The model under review builds one solid part; all positions refer to its coordinate system, in mm. Round coordinates to 2 decimals unless told otherwise and drop trailing zeros. Write each loop counter-clockwise with the first axis right and the second up, starting at its lowest first coordinate (ties: lowest second). Pieces come first, ordered by that corner, then holes. Notation, with made-up numbers: (-15, 3.25) -> (20, 3.25) arc R18 ccw to (20, 29.25) -> close; hole circle Ø1 at (-21, 54.25). An arc over 180 degrees is marked (long way). Return JSON: item names as keys, results as strings. Group by question number.
1. Clearance check with flat-ended pins moving along their axes: P1, Ø1.5, axis at x = -53, z = 4.5, coming from the +Y side; P2, Ø3, axis at x = 20.5, z = 9, coming from the +Y side; P3, Ø3, axis at y = -53, z = 6.5, coming from the +X side. State where each tip first meets the part, or that it passes through.
2. Take a section at B-B, the plane y = 5. Write out the cut boundary in (x, z).
3. Take a section at D-D, the plane x = 5. Write out the cut boundary in (y, z), then the cut area to 3 significant figures.
4. Take a section at A-A, the plane x = -52.5. Write out the cut boundary in (y, z), then the cut area to 3 significant figures.
5. Take a section at C-C, the plane y = -51. Write out the cut boundary in (x, z).
6. For line 1 along X through (y, z) = (42.5, 5); line 2 along X through (y, z) = (0.5, 4.75); line 3 along Z through (x, y) = (52.5, -45.25), list the stretches that pass through material, from the lowest coordinate up. Write a range as from..to.
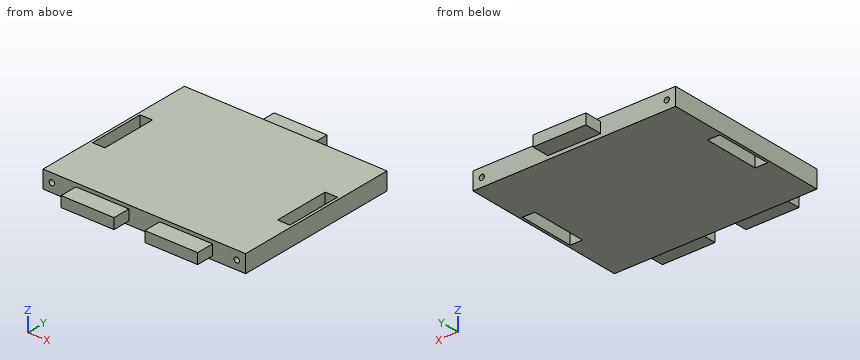
from build123d import *

# Parameters (mm, degrees)
ESBO_O1_W                = 115
ESBO_O1_H                = 95
RESSALTO_EXTRUS_O1_DEPTH = 10
ESBO_O2_W                = 30
ESBO_O2_H                = 6
RESSALTO_EXTRUS_O2_DEPTH = 10
ESBO_O3_W                = 30
ESBO_O3_H                = 6
RESSALTO_EXTRUS_O3_DEPTH = 10
ESBO_O4_W                = 7
ESBO_O4_H                = 32
CORTE_EXTRUS_O1_DEPTH    = 11
ESBO_O5_R                = 1.5
CORTE_EXTRUS_O2_DEPTH    = 8
ESBO_O6_R                = 1.5
CORTE_EXTRUS_O3_DEPTH    = 8


with BuildPart() as part:
    # Esboço1 → Ressalto-extrusão1 (new body)
    with BuildSketch(Plane.XY):
        Rectangle(ESBO_O1_W, ESBO_O1_H)
    extrude(amount=RESSALTO_EXTRUS_O1_DEPTH)

    # Esboço2 → Ressalto-extrusão2 (add)
    with BuildSketch(Plane(origin=(0, 47.5, 0), x_dir=(1, 0, 0), z_dir=(0, 1, 0))):
        with Locations((0, -5)):
            Rectangle(ESBO_O2_W, ESBO_O2_H)
    extrude(amount=RESSALTO_EXTRUS_O2_DEPTH)

    # Esboço3 → Ressalto-extrusão3 (add)
    with BuildSketch(Plane.XZ.offset(47.5)):
        with Locations((23.75, 5)):
            Rectangle(ESBO_O3_W, ESBO_O3_H)
        with Locations((-23.75, 5)):
            Rectangle(ESBO_O3_W, ESBO_O3_H)
    extrude(amount=RESSALTO_EXTRUS_O3_DEPTH)

    # Esboço4 → Corte-extrusão1 (cut, through all)
    with BuildSketch(Plane.XY.offset(10)):
        with Locations((-52.5, 0)):
            Rectangle(ESBO_O4_W, ESBO_O4_H)
        with Locations((52.5, 0)):
            Rectangle(ESBO_O4_W, ESBO_O4_H)
    extrude(amount=-CORTE_EXTRUS_O1_DEPTH, mode=Mode.SUBTRACT)

    # Esboço5 → Corte-extrusão2 (cut)
    with BuildSketch(Plane(origin=(0, 47.5, 0), x_dir=(1, 0, 0), z_dir=(0, 1, 0))):
        with Locations((52.5, -5)):
            Circle(ESBO_O5_R)
        with Locations((-52.5, -5)):
            Circle(ESBO_O5_R)
    extrude(amount=-CORTE_EXTRUS_O2_DEPTH, mode=Mode.SUBTRACT)

    # Esboço6 → Corte-extrusão3 (cut)
    with BuildSketch(Plane.XZ.offset(47.5)):
        with Locations((-52.5, 5)):
            Circle(ESBO_O6_R)
        with Locations((52.5, 5)):
            Circle(ESBO_O6_R)
    extrude(amount=-CORTE_EXTRUS_O3_DEPTH, mode=Mode.SUBTRACT)


solid = part.part
Output:
{
 "1": {"P1": "stops at y = 39.5", "P2": "stops at y = 47.5", "P3": "stops at x = 38.75"},
 "2": {"outline": "(-57.5, 0) -> (-56, 0) -> (-56, 10) -> (-57.5, 10) -> close; (-49, 0) -> (49, 0) -> (49, 10) -> (-49, 10) -> close; (56, 0) -> (57.5, 0) -> (57.5, 10) -> (56, 10) -> close"},
 "3": {"outline": "(-47.5, 0) -> (47.5, 0) -> (47.5, 2) -> (57.5, 2) -> (57.5, 8) -> (47.5, 8) -> (47.5, 10) -> (-47.5, 10) -> close", "area": "1,010 mm^2"},
 "4": {"outline": "(-47.5, 0) -> (-16, 0) -> (-16, 10) -> (-47.5, 10) -> (-47.5, 6.5) -> (-39.5, 6.5) -> (-39.5, 3.5) -> (-47.5, 3.5) -> close; (16, 0) -> (47.5, 0) -> (47.5, 3.5) -> (39.5, 3.5) -> (39.5, 6.5) -> (47.5, 6.5) -> (47.5, 10) -> (16, 10) -> close", "area": "582 mm^2"},
 "5": {"outline": "(-38.75, 2) -> (-8.75, 2) -> (-8.75, 8) -> (-38.75, 8) -> close; (8.75, 2) -> (38.75, 2) -> (38.75, 8) -> (8.75, 8) -> close"},
 "6": {"line 1": "x = -57.5..-54, -51..51, 54..57.5", "line 2": "x = -57.5..-56, -49..49, 56..57.5", "line 3": "z = 0..3.5, 6.5..10"}
}
